Check sheet for the modelled part. Datum: model origin and axes. Units: mm. A direction names the side the tool comes from. Give positions to 0.01 mm unless a question says otherwise; leave off trailing zeros. Order: outer loops, then holes, each group sorted by start corner. A loop starts at its lowest first (then second) coordinate and runs counter-clockwise, first axis right, second up.
from build123d import *

# Parameters (mm, degrees)
SKETCH1_R           = 1.878
SKETCH1_R_2         = 4
BOSS_EXTRUDE1_DEPTH = 5
FILLET1_R           = 3
FILLET2_R           = 3
FILLET3_R           = 1
FILLET4_R           = 1


with BuildPart() as part:
    # Sketch1 → Boss-Extrude1 (new body)
    with BuildSketch(Plane.XY):
        with BuildLine():
            Line((0, -12.5), (-35, -12.5))
            Line((-35, -12.5), (-35, -9))
            Line((-35, -9), (-13.521844546, -9))
            Line((-13.521844546, -9), (-10.422570658, -6.900726112))
            ThreePointArc((-10.422570658, -6.900726112), (-11.641569013, -4.552347848), (-12.338962679, -2))
            Line((-12.338962679, -2), (-35, -2))
            Line((-35, -2), (-35, 1.5))
            Line((-35, 1.5), (-12.409673646, 1.5))
            ThreePointArc((-12.409673646, 1.5), (9.354143467, 8.291561976), (0, -12.5))
        make_face()
        with Locations((0, 8)):
            Circle(SKETCH1_R, mode=Mode.SUBTRACT)
        with Locations((8, 0)):
            Circle(SKETCH1_R, mode=Mode.SUBTRACT)
        with Locations((0, -8)):
            Circle(SKETCH1_R, mode=Mode.SUBTRACT)
        with Locations((-8, 0)):
            Circle(SKETCH1_R, mode=Mode.SUBTRACT)
        Circle(SKETCH1_R_2, mode=Mode.SUBTRACT)
    extrude(amount=BOSS_EXTRUDE1_DEPTH)

    # Chamfer1
    # the kernel refuses this chamfer: 6.874632774, 6 mm, written as the material it adds along each edge
    with BuildSketch(Plane(origin=(-12.409673646, 1.5, 0), x_dir=(-0.9997808942395764, -0.02093235566086501, 0), z_dir=(0, 0, 1))) as chamfer1_piece_1:
        with BuildLine():
            Line((6.161688618, 0), (-1.363052276, -3.796482939))
            Line((-1.363052276, -3.796482939), (-1.486883786, -3.736733567))
            ThreePointArc((-1.486883786, -3.736733567), (-0.576736398, -1.931017764), (-0.136123845, 0.019352752))
            Line((-0.136123845, 0.019352752), (0.002878045, 0.13746253))
            ThreePointArc((0.002878045, 0.13746253), (3.082372441, 0.072987331), (6.164566664, 0.13746253))
            Line((6.164566664, 0.13746253), (6.161688618, 0))
        make_face()
    extrude(amount=5)

    # Fillet1
    fillet1_edges = [part.edges().sort_by_distance(p)[0] for p in [
        (-13.521844546, -9, 2.5),
        (-10.422570658, -6.900726112, 2.5),
        (-12.338962679, -2, 2.5),
    ]]
    fillet(fillet1_edges, radius=FILLET1_R)

    # Fillet2
    fillet2_edges = [part.edges().sort_by_distance(p)[0] for p in [
        (-18.327151282, 1.5, 2.5),
        (-11.369250275, 5.195204345, 2.5),
    ]]
    fillet(fillet2_edges, radius=FILLET2_R)

    # Fillet3
    fillet3_edges = [part.edges().sort_by_distance(p)[0] for p in [
        (-35, -2, 2.5),
        (-35, -9, 2.5),
    ]]
    fillet(fillet3_edges, radius=FILLET3_R)

    # Fillet4
    fillet4_edges = [part.edges().sort_by_distance(p)[0] for p in [
        (-35, 1.5, 2.5),
        (-35, -12.5, 2.5),
    ]]
    fillet(fillet4_edges, radius=FILLET4_R)


solid = part.part
1) Section check C-C, the plane z = 2.15. Record the cut outline in (x, y).
Recorded:
outline: (-35, -11.5) arc R1 ccw to (-34, -12.5) - (0, -12.5) arc R12.5 ccw (long way) to (-10.99, 5.96) arc R3 cw to (-12.21, 4.75) - (-17.67, 1.85) arc R3 cw to (-19.07, 1.5) - (-34, 1.5) arc R1 ccw to (-35, 0.5) - (-35, -1) arc R1 ccw to (-34, -2) - (-14.67, -2) arc R3 cw to (-11.83, -4.03) arc R12.5 ccw to (-11.55, -4.77) arc R3 cw to (-12.64, -8.4) - (-12.76, -8.48) arc R3 cw to (-14.44, -9) - (-34, -9) arc R1 ccw to (-35, -10) - close; hole circle Ø3.76 at (-8, 0); hole circle Ø8 at (0, 0); hole circle Ø3.76 at (0, -8); hole circle Ø3.76 at (0, 8); hole circle Ø3.76 at (8, 0)
2) Depth check by flat-ended pin: pin 1 Ø1.5 at (x, z) = (-26, 3) entering from +Y; pin 2 Ø3.5 at (x, y) = (8, 0) entering from -Z; pin 3 Ø2 at (x, z) = (-9, 2) entering from +Y. Enter the tip coordinate at first touch or a pass-through.
Recorded:
pin 1: stops at y = 1.5
pin 2: passes through
pin 3: stops at y = 9.6
3) Draft check along Y on faces 3 (the face through (-0.244, 9.862, 2.465)), 4 (the face through (-17, -12.5, 2)), 5 (the face through (-0.244, -6.138, 2.465)), 6 (the face through (-27, 1.5, 2)). Enter one of: +Y half, -Y half, draft (parallel to the pull), parting line (faces both ways), or undercut.
Recorded:
face 3: undercut
face 4: -Y half
face 5: undercut
face 6: +Y half
4) Set-up check for faces 1 (the face through (-24, -2, 2)), 2 (the face through (-35, -11, 2)): record each of +Z, -Z, +X, -X, +Y, -Y from which the full face is reachable in a straight line by a thin tool's end or side.
Recorded:
face 1: +Z, -Z, -X
face 2: +Z, -Z, -X, +Y, -Y
5) Section check A-A, the plane y = 0. Record the cut outline in (x, z).
Recorded:
outline: (-35, 0) - (-9.88, 0) - (-9.88, 5) - (-35, 5) - close; (-6.12, 0) - (-4, 0) - (-4, 5) - (-6.12, 5) - close; (4, 0) - (6.12, 0) - (6.12, 5) - (4, 5) - close; (9.88, 0) - (12.5, 0) - (12.5, 5) - (9.88, 5) - close
6) Material ranges on L1, parallel to Y at x = -25, z = 3.05; L2, parallel to X at y = -1.25, z = 4.8; L3, parallel to Y at x = -16, z = 3.35, recorded low to high.
Recorded:
L1: y = -12.5 to -9, -2 to 1.5
L2: x = -34.97 to -9.4, -6.6 to -3.8, 3.8 to 6.6, 9.4 to 12.44
L3: y = -12.5 to -9, -2 to 2.74
7) Section check D-D, the plane y = 2.75. Record the cut outline in (x, z), then the cut area to 3 significant figures.
Recorded:
outline: (-15.97, 0) - (-2.9, 0) - (-2.9, 5) - (-15.97, 5) - close; (2.9, 0) - (12.19, 0) - (12.19, 5) - (2.9, 5) - close
area: 112 mm2
8) Section check B-B, the plane x = -9. Record the cut outline in (y, z), then the cut area to 3 significant figures.
Recorded:
outline: (-12.5, 0) - (-1.59, 0) - (-1.59, 5) - (-12.5, 5) - close; (1.59, 0) - (8.67, 0) - (8.67, 5) - (1.59, 5) - close
area: 90.0 mm2
